Here's how the part is built. I have some questions about the finished solid (model axes, mm). Face numbers are marked on the shaded views. A direction names the side the tool comes from. Round coordinates to 2 decimals unless told otherwise and drop trailing zeros. Loops run counter-clockwise (first coordinate to the right, second up) from the corner with the lowest first, then second, coordinate; pieces in that order, holes last. Notation, with made-up numbers: M -5,66.25 L 29,66.25 A20 cw 29,91.25 Z; hole C -23,6.25 d1. An arc over 180 degrees is marked long. Answer as a JSON object with one key per item and string values.
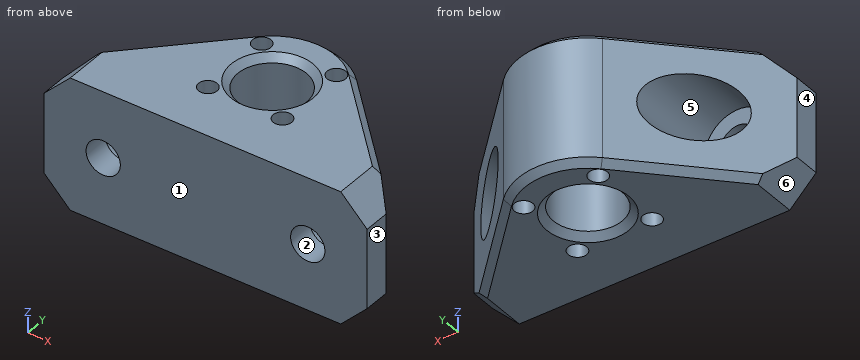
from build123d import *

# Parameters (mm, degrees)
PAD_DEPTH       = 20
SKETCH001_R     = 2.6
POCKET_DEPTH    = 24.501
SKETCH002_R     = 5
POCKET001_DEPTH = 20.501
SKETCH003_R     = 5.2
SKETCH003_R_2   = 1.4
POCKET002_DEPTH = 20.001
CHAMFER_SIZE    = 4
CHAMFER001_SIZE = 1
CHAMFER002_SIZE = 1


with BuildPart() as part:
    # Sketch → Pad (new body)
    with BuildSketch(Plane.XY):
        with BuildLine():
            Line((-24.5, 4), (-24.5, 0))
            Line((-24.5, 0), (24.5, 0))
            Line((24.5, 0), (24.5, 4))
            Line((7.499559, 21.348919), (24.5, 4))
            ThreePointArc((7.499559, 21.348919), (0, 24.5), (-7.499559, 21.348919))
            Line((-24.5, 4), (-7.499559, 21.348919))
        make_face()
    extrude(amount=PAD_DEPTH)

    # Sketch001 → Pocket (cut, through all)
    with BuildSketch(Plane.XZ):
        with Locations((-15.5, 10)):
            Circle(SKETCH001_R)
        with Locations((15.5, 10)):
            Circle(SKETCH001_R)
    extrude(amount=-POCKET_DEPTH, mode=Mode.SUBTRACT)

    # Sketch002 (on DatumPlane) → Pocket001 (cut, through all)
    with BuildSketch(Plane.XZ.offset(-4)):
        with Locations((-15.5, 10)):
            Circle(SKETCH002_R)
        with Locations((15.5, 10)):
            Circle(SKETCH002_R)
    extrude(amount=-POCKET001_DEPTH, mode=Mode.SUBTRACT)

    # Sketch003 → Pocket002 (cut, through all)
    with BuildSketch(Plane.XY):
        with Locations((0, 14)):
            Circle(SKETCH003_R)
        with Locations((-5.656854, 19.656854)):
            Circle(SKETCH003_R_2)
        with Locations((5.656854, 19.656854)):
            Circle(SKETCH003_R_2)
        with Locations((5.656854, 8.343146)):
            Circle(SKETCH003_R_2)
        with Locations((-5.656854, 8.343146)):
            Circle(SKETCH003_R_2)
    extrude(amount=POCKET002_DEPTH, mode=Mode.SUBTRACT)

    # Chamfer
    chamfer_edges = [part.edges().sort_by_distance(p)[0] for p in [
        (24.5, 2, 20),
        (24.5, 2, 0),
        (-24.5, 2, 20),
        (-24.5, 2, 0),
    ]]
    chamfer(chamfer_edges, length=CHAMFER_SIZE)

    # Chamfer001
    chamfer001_edges = [part.edges().sort_by_distance(p)[0] for p in [
        (-5.2, 14, 20),
        (-5.2, 14, 0),
    ]]
    chamfer(chamfer001_edges, length=CHAMFER001_SIZE)

    # Chamfer002
    chamfer002_edges = [part.edges().sort_by_distance(p)[0] for p in [
        (13.999779, 14.715456, 20),
        (0, 24.5, 20),
        (-13.999779, 14.715456, 20),
        (-13.999779, 14.715456, 0),
        (0, 24.5, 0),
        (13.999779, 14.715456, 0),
    ]]
    chamfer(chamfer002_edges, length=CHAMFER002_SIZE)


solid = part.part
Item 1: I want a section at C-C, the plane x = 0. Please give me the cut outline in (y, z).
Resolved:
{"outline": "M 0,0 L 7.8,0 L 8.8,1 L 8.8,19 L 7.8,20 L 0,20 Z; M 19.2,1 L 20.2,0 L 23.5,0 L 24.5,1 L 24.5,19 L 23.5,20 L 20.2,20 L 19.2,19 Z"}
Item 2: If we mould it in two halves opening along X, with no side actions, what happens to the marked faces 1, 2, 3 and 4? For each: pulls with the +X half, pulls with the -X half, needs draft (parallel to the pull), parting line crosses it, or undercut.
Resolved:
{"face 1": "needs draft", "face 2": "undercut", "face 3": "pulls with the +X half", "face 4": "pulls with the -X half"}
Item 3: I want a section at A-A, the plane z = 10. Please give me the cut outline in (x, y), then the cut area to 3 significant figures.
Resolved:
{"outline": "M -24.5,0 L -18.1,0 L -18.1,4 L -20.5,4 L -20.5,8.08 L -24.5,4 Z; M -12.9,0 L 12.9,0 L 12.9,4 L 10.5,4 L 10.5,18.29 L 7.5,21.35 A10.5 ccw -7.5,21.35 L -10.5,18.29 L -10.5,4 L -12.9,4 Z; M 18.1,0 L 24.5,0 L 24.5,4 L 20.5,8.08 L 20.5,4 L 18.1,4 Z; hole C -5.66,8.34 d2.8; hole C -5.66,19.66 d2.8; hole C 0,14 d10.4; hole C 5.66,8.34 d2.8; hole C 5.66,19.66 d2.8", "area": "449 mm²"}
Item 4: I'm going to push flat-ended pins straight in: pin 1 Ø1 at (x, z) = (-12.5, 11) entering from +Y; pin 2 Ø8 at (x, z) = (16, 12) entering from +Y; pin 3 Ø6 at (y, z) = (16, 17.5) entering from +X. Where does each tip first touch, or does it pass through?
Resolved:
{"pin 1": "y = 4", "pin 2": "y = 16.18", "pin 3": "x = 15.68"}
Item 5: I want a section at B-B, the plane y = 1.5. Please give me the cut outline in (x, z).
Resolved:
{"outline": "M -24.5,4 L -20.5,0 L 20.5,0 L 24.5,4 L 24.5,16 L 20.5,20 L -20.5,20 L -24.5,16 Z; hole C -15.5,10 d5.2; hole C 15.5,10 d5.2"}
Item 6: Please list where these lines run through material, in increasing order: probe 1 along X at (y, z) = (19.75, 13.5); probe 2 along Z at (x, y) = (15.5, 1.3); probe 3 along X at (y, z) = (19.25, 15.25). Write a range as from..to.
Resolved:
{"probe 1": "-9.07..-7.05, -4.26..4.26, 7.05..9.07", "probe 2": "0..7.4, 12.6..20", "probe 3": "-9.56..-7, -4.32..4.32, 7..9.56"}
Item 7: On a 3-axis mill with a long thin cutter (end or side, diameter ignored), from which of +Z, -Z, +X, -X, +Y, -Y can I reach the whole of each face in a straight line? I mean the marked faces 5 and 6. Say none if no direction works.
Resolved:
{"face 5": "+Y", "face 6": "-Z, -X, +Y, -Y"}
Item 8: I want a section at D-D, the plane z = 15.5. Please give me the cut outline in (x, y), then the cut area to 3 significant figures.
Resolved:
{"outline": "M -24.5,0 L 24.5,0 L 24.5,4 L 7.5,21.35 A10.5 ccw -7.5,21.35 L -24.5,4 Z; hole C -5.66,8.34 d2.8; hole C -5.66,19.66 d2.8; hole C 0,14 d10.4; hole C 5.66,8.34 d2.8; hole C 5.66,19.66 d2.8", "area": "674 mm²"}
